The model under review builds one solid part; all positions refer to its coordinate system, in mm. A direction names the side the tool comes from. Coordinates: 2 decimals unless noted, no trailing zeros. Loops run counter-clockwise (first coordinate to the right, second up) from the corner with the lowest first, then second, coordinate; pieces in that order, holes last. Notation, with made-up numbers: M 35,1.5 L 92,1.5 A22 cw 92,38.5 Z; hole C 89.25,-38 d8. An arc over 180 degrees is marked long. Write item = value, one per line. Start each with the question number.
Q1. We need section D-D on x = 13. Give the boundary of the cut face in (y, z), and give its area (3 significant figures).
Q2. We need section B-B on x = 52. Give the boundary of the cut face in (y, z), and give its area (3 significant figures).
Q3. We need section C-C on y = 25.5. Give the boundary of the cut face in (x, z).
Q4. For faces 1 (the face through (-25, -31.895, 12)), 2 (the face through (7, 51.105, 12)), 3 (the face through (24, 21.105, 12)), list the 3-axis set-ups (+Z, -Z, +X, -X, +Y, -Y) from which the entire face can be reached by the end or side of a thin tool; tool diameter is ignored.
Q5. We need section A-A on z = 2.25. Give the boundary of the cut face in (x, y).
Q6. Mouldability with a two-part tool opening along X and no side actions: class faces 4 (the face through (-55.511, 10, 12)), 5 (the face through (28.618, -31.065, 12.325)), 6 (the face through (6, 12, 25)) as released by +X, released by -X, zero draft, split by the parting line, or undercut.
Q7. Clearance check with flat-ended pins moving along their axes: pin 1 Ø5 at (x, z) = (12.5, 3.5) entering from -Y; pin 2 Ø4 at (x, z) = (-30.5, 17) entering from -Y; pin 3 Ø2.5 at (y, z) = (-49, 18) entering from -X. State where each tip first meets the part, or that it passes through.
Q8. Wall thickness on probe 1 along Y at (x, z) = (44, 5.75); probe 2 along Y at (x, z) = (-7, 11.75); probe 3 along X at (y, z) = (-15.5, 22): over which ranges is each line inside the solid? List them lowest first.
from build123d import *

# Parameters (mm, degrees)
F0_R     = 20
F1_DEPTH = 25


with BuildPart() as f1:
    # F0 (on Top) → F1 (new body)
    with BuildSketch(Plane.XY):
        with Locations((44.489244, -18.895161)):
            Circle(F0_R)
        with BuildLine():
            ThreePointArc((-15.510756, -13.895161), (-32.581823, -6.824093), (-25.510756, -23.895161))
            ThreePointArc((-25.510756, -23.895161), (-18.439688, -20.966228), (-15.510756, -13.895161))
        make_face()
        with BuildLine():
            Line((21.489244, -51.895161), (68.489244, -51.895161))
            Line((68.489244, -51.895161), (68.489244, -18.895161))
            Line((68.489244, -18.895161), (68.489244, 51.104839))
            Line((68.489244, 51.104839), (63.193549, 51.104839))
            Line((63.193549, 51.104839), (-55.510756, 51.104839))
            Line((-55.510756, 51.104839), (-55.510756, -31.895161))
            Line((-55.510756, -31.895161), (-25.510756, -31.895161))
            Line((-25.510756, -31.895161), (6.489244, -31.895161))
            ThreePointArc((6.489244, -31.895161), (17.095846, -36.288559), (21.489244, -46.895161))
            Line((21.489244, -46.895161), (21.489244, -51.895161))
        make_face()
        with BuildLine():
            ThreePointArc((-15.510756, -13.895161), (-18.439688, -20.966228), (-25.510756, -23.895161))
            ThreePointArc((-25.510756, -23.895161), (-32.581823, -6.824093), (-15.510756, -13.895161))
        make_face(mode=Mode.SUBTRACT)
        with Locations((44.489244, -18.895161)):
            Circle(F0_R, mode=Mode.SUBTRACT)
        with BuildLine():
            ThreePointArc((63.193549, 29.104839), (60.850403, 23.447985), (55.193549, 21.104839))
            Line((55.193549, 21.104839), (-7.806451, 21.104839))
            ThreePointArc((-7.806451, 21.104839), (-13.463306, 23.447985), (-15.806451, 29.104839))
            ThreePointArc((-15.806451, 29.104839), (-13.463306, 34.761694), (-7.806451, 37.104839))
            Line((-7.806451, 37.104839), (55.193549, 37.104839))
            ThreePointArc((55.193549, 37.104839), (60.850403, 34.761694), (63.193549, 29.104839))
        make_face(mode=Mode.SUBTRACT)
    extrude(amount=F1_DEPTH)


solid = f1.part
Returned:
q1.outline = M -33.38,0 L 21.1,0 L 21.1,25 L -33.38,25 Z; M 37.1,0 L 51.1,0 L 51.1,25 L 37.1,25 Z
q1.area = 1,710 mm^2
q2.outline = M -51.9,0 L -37.43,0 L -37.43,25 L -51.9,25 Z; M -0.36,0 L 21.1,0 L 21.1,25 L -0.36,25 Z; M 37.1,0 L 51.1,0 L 51.1,25 L 37.1,25 Z
q2.area = 1,250 mm^2
q3.outline = M -55.51,0 L -14.95,0 L -14.95,25 L -55.51,25 Z; M 62.34,0 L 68.49,0 L 68.49,25 L 62.34,25 Z
q4.face_1 = +Z, -Z, -X, -Y
q4.face_2 = +Z, -Z, +X, -X, +Y
q4.face_3 = +Z, -Z
q5.outline = M -55.51,-31.9 L 6.49,-31.9 A15 cw 21.49,-46.9 L 21.49,-51.9 L 68.49,-51.9 L 68.49,51.1 L -55.51,51.1 Z; hole M -25.51,-23.9 A10 ccw -15.51,-13.9 A10 ccw long Z; hole M -15.81,29.1 A8 ccw -7.81,21.1 L 55.19,21.1 A8 ccw 63.19,29.1 A8 ccw 55.19,37.1 L -7.81,37.1 A8 ccw Z; hole C 44.49,-18.9 d40
q6.face_4 = released by -X
q6.face_5 = undercut
q6.face_6 = zero draft
q7.pin_1 = -34.54
q7.pin_2 = -31.9
q7.pin_3 = 21.49
q8.probe_1 = -51.9 to -38.89, 1.1 to 21.1, 37.1 to 51.1
q8.probe_2 = -31.9 to 21.1, 37.1 to 51.1
q8.probe_3 = -55.51 to -35.38, -15.64 to 24.78, 64.2 to 68.49
